Read the model definition and answer for the solid it produces. Units are mm, in the model's axes. A direction names the side the tool comes from. Give positions to 0.01 mm unless a question says otherwise; leave off trailing zeros. Order: outer loops, then holes, each group sorted by start corner. A loop starts at its lowest first (then second) coordinate and runs counter-clockwise, first axis right, second up. Notation, with made-up numbers: (-1, 62.5) - (24, 62.5) arc R28 cw to (24, 91.5) - close; hole circle Ø11 at (60, 63). An arc over 180 degrees is marked (long way). Write each question's results on one line, items separated by ' | '.
from build123d import *

# Parameters (mm, degrees)
F0_W     = 101.6
F0_H     = 101.6
F0_W_2   = 76.2
F0_H_2   = 76.2
F1_DEPTH = 203.2
F2_SIZE  = 12.7
F3_SIZE  = 12.7


with BuildPart() as f1:
    # F0 (on Top) → F1 (new body)
    with BuildSketch(Plane.XY):
        with Locations((50.8, 50.8)):
            Rectangle(F0_W, F0_H)
        with Locations((50.8, 50.8)):
            Rectangle(F0_W_2, F0_H_2, mode=Mode.SUBTRACT)
    extrude(amount=F1_DEPTH)

    # F2
    f2_edges = [f1.edges().sort_by_distance(p)[0] for p in [
        (12.7, 88.9, 101.6),
        (88.9, 88.9, 101.6),
        (88.9, 12.7, 101.6),
        (12.7, 12.7, 101.6),
    ]]
    chamfer(f2_edges, length=F2_SIZE)

    # F3
    f3_edges = [f1.edges().sort_by_distance(p)[0] for p in [
        (101.6, 0, 101.6),
        (101.6, 101.6, 101.6),
        (0, 0, 101.6),
        (0, 101.6, 101.6),
    ]]
    chamfer(f3_edges, length=F3_SIZE)


solid = f1.part
(1) For faces 1 (the face through (82.6, 19.1, 100.2)), 2 (the face through (6.4, 6.3, 100.2)), determine the directions among +Z, -Z, +X, -X, +Y, -Y from which every point of the face is accessible in a straight line to the end or side of a thin tool.
Conclusion:
face 1: +Z, -Z | face 2: +Z, -Z, -X, -Y
(2) This flat-tipped pin is pushed along its axis until it touches: pin 1 (4 mm diameter, centred on x = 12, z = 157, fed in from +Y). Where does it stop, or does it pass through?
Conclusion:
pin 1: y = 101.6
(3) Section C-C (z = 13.5) is taken. Give the vertices of the cut face in (x, y), plus the area to 3 significant figures.
Conclusion:
outline: (0, 12.7) - (12.7, 0) - (88.9, 0) - (101.6, 12.7) - (101.6, 88.9) - (88.9, 101.6) - (12.7, 101.6) - (0, 88.9) - close; hole (12.7, 25.4) - (25.4, 12.7) - (76.2, 12.7) - (88.9, 25.4) - (88.9, 76.2) - (76.2, 88.9) - (25.4, 88.9) - (12.7, 76.2) - close | area: 4,520 mm^2
(4) Section D-D (y = 6) is taken. Give the vertices of the cut face in (x, z).
Conclusion:
outline: (6.7, 0) - (94.9, 0) - (94.9, 203.2) - (6.7, 203.2) - close
(5) The mould has two halves that part along X. Classify faces 3 (the face through (95.3, 95.2, 100.2)), 4 (the face through (82.5, 82.6, 100.2)), 5 (the face through (88.9, 50, 100)), 6 (the face through (50, 0, 100)): pulls with the +X half, pulls with the -X half, needs draft (parallel to the pull), parting line crosses it, or undercut.
Conclusion:
face 3: pulls with the +X half | face 4: undercut | face 5: undercut | face 6: needs draft
(6) Section A-A (x = 62.5) is taken. Give the vertices of the cut face in (y, z), plus the area to 3 significant figures.
Conclusion:
outline: (0, 0) - (12.7, 0) - (12.7, 203.2) - (0, 203.2) - close; (88.9, 0) - (101.6, 0) - (101.6, 203.2) - (88.9, 203.2) - close | area: 5,160 mm^2
(7) Consider probe 1 along X at (y, z) = (68, 112); probe 2 along X at (y, z) = (20.5, 73). Determine where each line is inside the solid, lowest interval first. Write a range as [from, to].
Conclusion:
probe 1: [0, 12.7], [88.9, 101.6] | probe 2: [0, 17.6], [84, 101.6]
